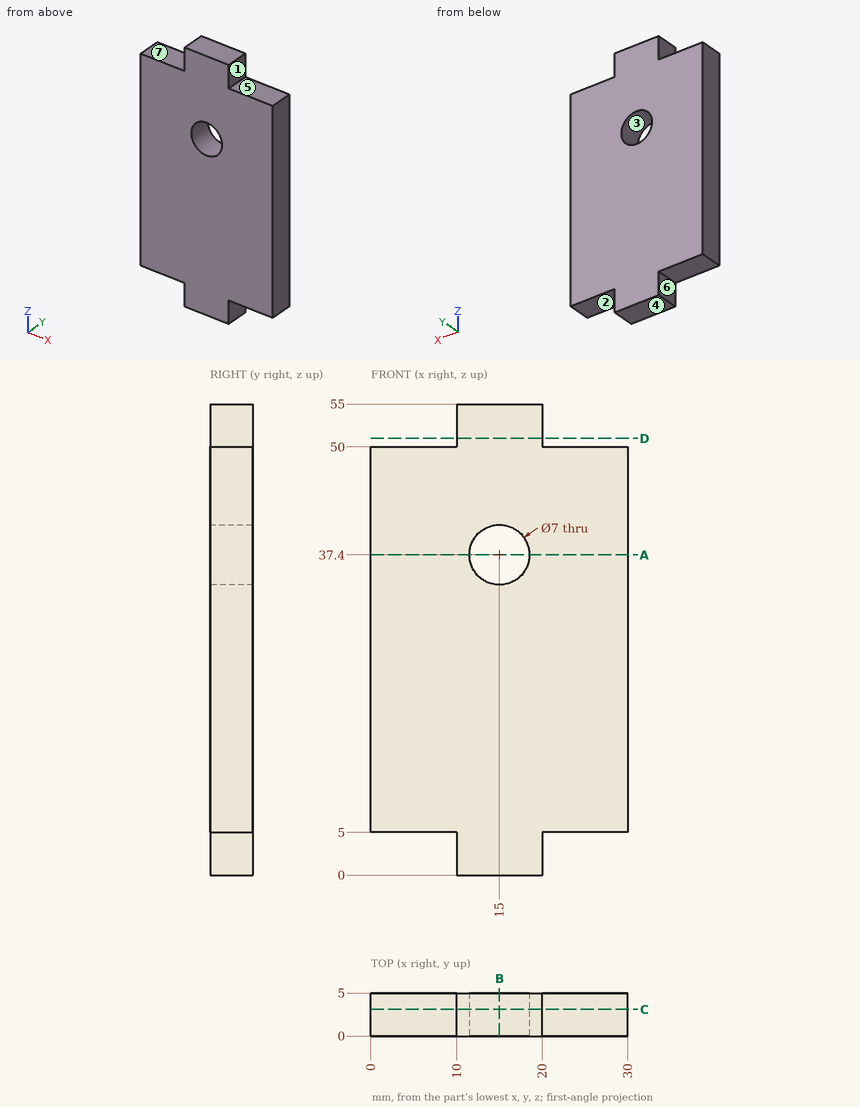
Part print with two shaded views. Sizes in mm from the minimum x, y, z corner. A direction names the side the tool comes from. Round coordinates to 2 decimals unless told otherwise and drop trailing zeros. Order: outer loops, then holes, each group sorted by start corner. A loop starts at its lowest first (then second) coordinate and runs counter-clockwise, first axis right, second up. Notation, with made-up numbers: M 79.25,3 L 138.25,3 A19 ccw 138.25,22 Z; hole C 26.5,20 d8. An arc over 180 degrees is marked long. Put each result on its own line as item: value. Start each with the question number.
1. Drill centre lines: probe 1 along X at (y, z) = (2.55, 37.4); probe 2 along Z at (x, y) = (25, 2.85); probe 3 along X at (y, z) = (2.25, 53.5). Where is each one in solid material? Low to high. Write a range as [from, to].
2. Slice it at D-D on z = 51. List the corners of the cut face in (x, y).
3. Slice it at B-B on x = 15. List the corners of the cut face in (y, z).
4. Two-plate mould, pull along X, no slides. Class the marked faces 1, 2 and 3: +X half, -X half, draft (parallel to the pull), parting line (faces both ways), or undercut.
5. Slice it at A-A on z = 37.4. List the corners of the cut face in (x, y), then the cut area to 3 significant figures.
6. Drop flat-ended pins along their axis: pin 1 (1.5 mm diameter, centred on x = 5.5, y = 3.5, fed in from -Z); pin 2 (2.5 mm diameter, centred on y = 3.5, z = 53.5, fed in from +X). Give the stop position or say it passes through.
7. Tool access for the marked faces 4, 5, 6 and 7: list every direction of +Z, -Z, +X, -X, +Y, -Y with a clear straight run to the whole face (end or side of a thin tool).
8. Slice it at C-C on y = 3.1. List the corners of the cut face in (x, z), then the cut area to 3 significant figures.
Findings:
1. probe 1: [0, 11.5], [18.5, 30]
1. probe 2: [5, 50]
1. probe 3: [10, 20]
2. outline: M 10,0 L 20,0 L 20,5 L 10,5 Z
3. outline: M 0,0 L 5,0 L 5,33.9 L 0,33.9 Z; M 0,40.9 L 5,40.9 L 5,55 L 0,55 Z
4. face 1: +X half
4. face 2: draft
4. face 3: undercut
5. outline: M 0,0 L 11.5,0 L 11.5,5 L 0,5 Z; M 18.5,0 L 30,0 L 30,5 L 18.5,5 Z
5. area: 115 mm2
6. pin 1: z = 5
6. pin 2: x = 20
7. face 4: -Z, +X, -X, +Y, -Y
7. face 5: +Z, +X, +Y, -Y
7. face 6: -Z, -X, +Y, -Y
7. face 7: +Z, -X, +Y, -Y
8. outline: M 0,5 L 10,5 L 10,0 L 20,0 L 20,5 L 30,5 L 30,50 L 20,50 L 20,55 L 10,55 L 10,50 L 0,50 Z; hole C 15,37.4 d7
8. area: 1,410 mm2
